from build123d import *

# Parameters (mm, degrees)
F0_W     = 38.1
F0_H     = 19.05
F1_DEPTH = 406.4
F2_R     = 5.08
F3_SIZE  = 5.08
F4_R     = 1.984375
F5_DEPTH = 25.4


with BuildPart() as f1:
    # F0 (on Right) → F1 (new body)
    with BuildSketch(Plane.YZ):
        with Locations((19.05, 9.525)):
            Rectangle(F0_W, F0_H)
    extrude(amount=F1_DEPTH)

    # F2
    f2_edges = [f1.edges().sort_by_distance(p)[0] for p in [
        (203.2, 0, 19.05),
        (203.2, 38.1, 19.05),
    ]]
    fillet(f2_edges, radius=F2_R)

    # F3
    f3_edges = [f1.edges().sort_by_distance(p)[0] for p in [
        (406.4, 19.05, 19.05),
        (0, 19.05, 19.05),
    ]]
    chamfer(f3_edges, length=F3_SIZE)

    # F4 (on face) → F5 (cut)
    with BuildSketch(Plane(origin=(0, 0, 0), x_dir=(1, 0, 0), z_dir=(0, 0, -1))):
        with Locations((31.75, -19.05)):
            Circle(F4_R)
        with Locations((374.65, -19.05)):
            Circle(F4_R)
    extrude(amount=-F5_DEPTH, mode=Mode.SUBTRACT)


solid = f1.part
Input: part model. Units: mm. Frame: model coordinates. Give positions to 0.01 mm unless a question says otherwise; leave off trailing zeros. Order: outer loops, then holes, each group sorted by start corner. A loop starts at its lowest first (then second) coordinate and runs counter-clockwise, first axis right, second up.
Q1. Contact query for flat-ended pins moving along their axis: pin 1 Ø2 at (x, y) = (331.5, 26) entering from -Z; pin 2 Ø3 at (x, y) = (31.75, 19.05) entering from -Z. Output: stop coordinate, or through.
Checked values:
pin 1: stops at z = 0
pin 2: passes through
Q2. Ray query, probe 1 along X at (y, z) = (19.05, 4.75); probe 2 along X at (y, z) = (18, 2); probe 3 along Y at (x, z) = (31.75, 7). Return the intervals inside material, ascending.
Checked values:
probe 1: x = 0 to 29.77, 33.73 to 372.67, 376.63 to 406.4
probe 2: x = 0 to 30.07, 33.43 to 372.97, 376.33 to 406.4
probe 3: y = 0 to 17.07, 21.03 to 38.1
Q3. Section A-A on x = 157.5. Output: boundary loops of the cut face in (y, z), and give its area (3 significant figures).
Checked values:
outline: (0, 0) - (38.1, 0) - (38.1, 13.97) arc R5.08 ccw to (33.02, 19.05) - (5.08, 19.05) arc R5.08 ccw to (0, 13.97) - close
area: 715 mm2
